Autodesk Fusion 360 part; units mm, degrees
sketch "Sketch1" plane through (0, 0, 0) normal (0, 0, 1) x (1, 0, 0) in component "ex2"
  circle A0 centre (0, 0) radius 30
  circle A1 centre (129, 0) radius 20
  line L0 (0, 0) -> (0, 43.8518) construction
  line L1 (129, 0) -> (129, 43.6821) construction
  line L2 (-11.547, 20) -> (-23.094, 0)
  line L3 (-23.094, 0) -> (-11.547, -20)
  line L4 (-11.547, -20) -> (11.547, -20)
  line L5 (11.547, -20) -> (23.094, 0)
  line L6 (23.094, 0) -> (11.547, 20)
  line L7 (11.547, 20) -> (-11.547, 20)
  line L8 (129, 15) -> (114.7342, 4.6353)
  line L9 (114.7342, 4.6353) -> (120.1832, -12.1353)
  line L10 (120.1832, -12.1353) -> (137.8168, -12.1353)
  line L11 (137.8168, -12.1353) -> (143.2658, 4.6353)
  line L12 (143.2658, 4.6353) -> (129, 15)
  line L13 (28.2843, 10) -> (111.6795, 10)
  line L14 (49.2985, 10) -> (49.2985, -10) construction
  line L15 (49.2985, 0) -> (56, 0) construction
  line L16 (28.2843, -10) -> (111.6795, -10)
  line L17 (119.4894, -10) -> (120.196, -10)
  line L18 (30, 0) -> (109, 0)
  line L19 (71.1993, 0) -> (71.1993, 28.9403) construction
  line L20 (101.1993, 5) -> (41.1993, 5)
  line L21 (41.1993, -5) -> (101.1993, -5)
  line L22 (101.1993, 5) -> (41.1993, -5) construction
  line L23 (41.1993, 5) -> (101.1993, -5) construction
  arc A2 (42.8209, 4.7297) -> (42.8209, -4.7297) centre (41.1993, 0) ccw
  arc A3 (99.5777, -4.7297) -> (99.5777, 4.7297) centre (101.1993, 0) ccw
  point P0 (129, 0)
  point P1 (71.1993, 0)
  dimension "d9" = 60
  dimension "d10" = 40
  dimension "d11" = 129
  dimension "d12" = 20
  dimension "d13" = 15
  dimension "d14" = 10
  dimension "d15" = 10
  dimension "d16" = 60
  dimension "d17" = 10
extrude "Extrude1" add sketch "Sketch1" along normal blind 10 contours A0 | A1 makes body 1 at (29.8509, 2.987, 6.6667) makes body 2 at (148.9006, -1.9914, 3.3333) in component "ex2"
extrude "Extrude2" add sketch "Sketch1" along normal mid plane 12 contours A0 A1 L16 L18 L21 A2 A3 | A0 A1 L13 L18 L20 A2 A3 bodies 1 2 in component "ex2"
extrude "Extrude3" add sketch "Sketch1" along normal mid plane 6 contours L18 L20 A2 A3 bodies 1 in component "ex2"
component "ex2" placed x (1, 0, 0) y (0, 1, 0) z (0, 0, 1) at (0, 0, 0)
Input: part model. Units: mm. Frame: model coordinates. A direction names the side the tool comes from. Round coordinates to 2 decimals unless told otherwise and drop trailing zeros. Loops run counter-clockwise (first coordinate to the right, second up) from the corner with the lowest first, then second, coordinate; pieces in that order, holes last. Notation, with made-up numbers: M 74.5,42.5 L 100.5,42.5 A25 ccw 100.5,72.5 Z; hole C -9.5,-30.75 d5. An arc over 180 degrees is marked long. Answer in a Markdown table with one row per item. Add a question column.
1. Section C-C (x = 125). Output: boundary loops of the cut face in (y, z).
2. Ray query, probe 1 along Y at (x, z) = (94, -0.25); probe 2 along X at (y, z) = (0, 3.25); probe 3 along X at (y, z) = (-13.5, 2). Return the intervals inside material, ascending.
3. Mould query, pull axis X, two halves, no side actions, for faces 1 (the face through (129, -13, 0)), 2 (the face through (109, 0, -3)), 3 (the face through (69, 7, 6)). Classes: released by +X, released by -X, zero draft, split by the parting line, or undercut.
4. Section A-A (x = 0). Output: boundary loops of the cut face in (y, z), and give its area (3 significant figures).
5. Section D-D (y = 26). Output: boundary loops of the cut face in (x, z).
6. Contact query for flat-ended pins moving along their axis: pin 1 (18 mm diameter, centred on x = 15, y = 1.5, fed in from -Z); pin 2 (6 mm diameter, centred on x = 56.5, z = 0.5, fed in from +Y); pin 3 (10 mm diameter, centred on x = 49.5, y = -4.5, fed in from +Z). Output: stop coordinate, or through.
7. Section B-B (x = 49). Output: boundary loops of the cut face in (y, z), and give its area (3 significant figures).
8. Set-up query: faces 4 (the face through (69, 10, 0)), 5 (the face through (69, -10, 0)), 6 (the face through (17.4, 9.86, 4.93)), 7 (the face through (71, 3, 3)). Return all of +Z, -Z, +X, -X, +Y, -Y with unobstructed straight access to the full face (end or side cutting, diameter ignored); none if empty.
Values follow:
| question | item | result |
|---|---|---|
| 1 | outline | M -19.6,0 L -12.14,0 L -12.14,10 L -19.6,10 Z; M 12.09,0 L 19.6,0 L 19.6,10 L 12.09,10 Z |
| 2 | probe 1 | -10 to -5, 0 to 10 |
| 2 | probe 2 | -30 to -23.09, 23.09 to 36.2, 106.2 to 116.24, 141.76 to 149 |
| 2 | probe 3 | -26.79 to -15.3, 15.3 to 26.79, 114.24 to 143.76 |
| 3 | face 1 | zero draft |
| 3 | face 2 | released by +X |
| 3 | face 3 | undercut |
| 4 | outline | M -30,0 L -20,0 L -20,10 L -30,10 Z; M 20,0 L 30,0 L 30,10 L 20,10 Z |
| 4 | area | 200 mm^2 |
| 5 | outline | M -14.97,0 L 14.97,0 L 14.97,10 L -14.97,10 Z |
| 6 | pin 1 | z = 0 |
| 6 | pin 2 | y = 10 |
| 6 | pin 3 | z = 6 |
| 7 | outline | M -10,-6 L -5,-6 L -5,6 L -10,6 Z; M 0,-3 L 5,-3 L 5,-6 L 10,-6 L 10,6 L 5,6 L 5,3 L 0,3 Z |
| 7 | area | 150 mm^2 |
| 8 | face 4 | +Z, -Z, +Y |
| 8 | face 5 | +Z, -Z, -Y |
| 8 | face 6 | +Z, -Z |
| 8 | face 7 | +Z |
